```python
from build123d import *

# Parameters (mm, degrees)
SKETCH1_W                       = 10.3124
SKETCH1_H                       = 15.1892
SKETCH1_R                       = 1.8669
BOSS_EXTRUDE1_DEPTH             = 1.27
BOSS_EXTRUDE2_REACH             = 15.485
BOSS_EXTRUDE2_DIRECTION_2_REACH = 15.485
BOSS_EXTRUDE3_DEPTH             = 0.4318
LPATTERN1_COUNT                 = 5
LPATTERN1_PITCH                 = 1.27
BOSS_EXTRUDE4_DEPTH             = 6.3754
BOSS_EXTRUDE5_DEPTH             = 11.1252
BOSS_EXTRUDE5_DEPTH_BACK        = 4.7752


with BuildPart() as part:
    # Sketch1 → Boss-Extrude1 (new body)
    with BuildSketch(Plane(origin=(0, 0, 0), x_dir=(1, 0, 0), z_dir=(0, 1, 0))):
        with Locations((0, -4.8006)):
            Rectangle(SKETCH1_W, SKETCH1_H)
        with Locations(Location((0, 0, 0), (0, 0, 270))):
            Circle(SKETCH1_R, mode=Mode.SUBTRACT)
    extrude(amount=BOSS_EXTRUDE1_DEPTH)

    # Boss-Extrude2: up to this face of the body (flat: up to its plane)
    boss_extrude2_end = Plane(part.part.faces().sort_by_distance((5.1562, 0.635, 4.8006))[0])
    # Sketch2 → Boss-Extrude2 (add, up to the picked face)
    with BuildSketch(Plane(origin=(0, 0, 0), x_dir=(0, 0, -1), z_dir=(1, 0, 0)), mode=Mode.PRIVATE) as boss_extrude2_sk1:
        Polygon((-3.302, 1.2192), (-3.906625217, 4.6482), (-12.32801942, 4.6482), (-12.663922319, 2.7432), (-12.3952, 1.2192), align=None)
    boss_extrude2_tool1 = split(extrude(boss_extrude2_sk1.sketch, amount=BOSS_EXTRUDE2_REACH, mode=Mode.PRIVATE), bisect_by=boss_extrude2_end, keep=Keep.BOTH, mode=Mode.PRIVATE)
    add(boss_extrude2_tool1.solids().sort_by(Axis((0, 2.911082, 8.056355), (1, 0, 0)))[0])

    # Boss-Extrude2 direction 2: up to this face of the body (flat: up to its plane)
    boss_extrude2_direction_2_end = Plane(part.part.faces().sort_by_distance((-5.1562, 0.635, 4.8006))[0])
    # Sketch2 → Boss-Extrude2 direction 2 (add, up to the picked face)
    with BuildSketch(Plane(origin=(0, 0, 0), x_dir=(0, 0, -1), z_dir=(1, 0, 0)), mode=Mode.PRIVATE) as boss_extrude2_direction_2_sk1:
        Polygon((-3.302, 1.2192), (-3.906625217, 4.6482), (-12.32801942, 4.6482), (-12.663922319, 2.7432), (-12.3952, 1.2192), align=None)
    boss_extrude2_direction_2_tool1 = split(extrude(boss_extrude2_direction_2_sk1.sketch, amount=-BOSS_EXTRUDE2_DIRECTION_2_REACH, mode=Mode.PRIVATE), bisect_by=boss_extrude2_direction_2_end, keep=Keep.BOTH, mode=Mode.PRIVATE)
    add(boss_extrude2_direction_2_tool1.solids().sort_by(Axis((0, 2.911082, 8.056355), (-1, 0, 0)))[0])

    # Sketch3 → Boss-Extrude3 (add, symmetric)
    with BuildSketch(Plane(origin=(2.54, 0, 0), x_dir=(0, 0, -1), z_dir=(1, 0, 0))):
        with BuildLine():
            Line((-11.1252, 2.54), (-18.7452, 2.54))
            ThreePointArc((-18.7452, 2.54), (-18.762931645, 2.540154742), (-18.780657889, 2.54061892))
            Line((-18.780657889, 2.54061892), (-25.050636059, 2.759571382))
            Line((-25.050636059, 2.759571382), (-25.032907115, 3.267261922))
            Line((-25.032907115, 3.267261922), (-18.762928944, 3.04830946))
            ThreePointArc((-18.762928944, 3.04830946), (-18.754065822, 3.048077371), (-18.7452, 3.048))
            Line((-18.7452, 3.048), (-11.1252, 3.048))
            Line((-11.1252, 3.048), (-11.1252, 2.54))
        make_face()
    boss_extrude3 = extrude(amount=BOSS_EXTRUDE3_DEPTH, both=True)

    # LPattern1: Boss-Extrude3 ×5
    with Locations(*[(-i * LPATTERN1_PITCH, 0, 0) for i in range(1, LPATTERN1_COUNT)]):
        add(boss_extrude3)

    # Sketch4 → Boss-Extrude4 (add, symmetric)
    with BuildSketch(Plane(origin=(0, 0, 0), x_dir=(0, 0, -1), z_dir=(1, 0, 0))):
        Polygon((-18.796, 0.5969), (-30.48, 0.5969), (-30.48, 6.8453), (-24.2316, 6.8453), (-24.2316, 4.7371), (-17.272, 4.7371), (-17.272, 1.3589), (-18.796, 1.3589), align=None)
    extrude(amount=BOSS_EXTRUDE4_DEPTH, both=True)

    # Sketch5 → Boss-Extrude5 (add, two sides: drawn at the far end of the back side and taken through both)
    with BuildSketch(Plane.XY.offset(-BOSS_EXTRUDE5_DEPTH_BACK)):
        with BuildLine():
            Line((5.715, 0), (-5.715, 0))
            ThreePointArc((-5.715, 0), (-6.368072211, 0.237698846), (-6.715564677, 0.839573451))
            Line((-6.715564677, 0.839573451), (-9.124737032, 14.502668828))
            Line((-9.124737032, 14.502668828), (-10.125301709, 14.326242279))
            Line((-10.125301709, 14.326242279), (-7.716129354, 0.663146903))
            ThreePointArc((-7.716129354, 0.663146903), (-7.021144423, -0.540602308), (-5.715, -1.016))
            Line((-5.715, -1.016), (5.715, -1.016))
            ThreePointArc((5.715, -1.016), (7.021144423, -0.540602308), (7.716129354, 0.663146903))
            Line((7.716129354, 0.663146903), (10.125301709, 14.326242279))
            Line((10.125301709, 14.326242279), (9.124737032, 14.502668828))
            Line((9.124737032, 14.502668828), (6.715564677, 0.839573451))
            ThreePointArc((6.715564677, 0.839573451), (6.368072211, 0.237698846), (5.715, 0))
        make_face()
    extrude(amount=BOSS_EXTRUDE5_DEPTH + BOSS_EXTRUDE5_DEPTH_BACK)


solid = part.part
```
Model file for the job. Use its own axes, mm. A direction names the side the tool comes from. Round coordinates to 2 decimals unless told otherwise and drop trailing zeros. Write each loop counter-clockwise with the first axis right and the second up, starting at its lowest first coordinate (ties: lowest second). Pieces come first, ordered by that corner, then holes. Notation, with made-up numbers: M 28,37.5 L 39,37.5 A11 ccw 39,41.5 Z; hole C 29.25,-27 d9. An arc over 180 degrees is marked long. Put each result on its own line as item: value.
Item 1: Mould opens along Z. For faces 6 (the flat face through (1, 3.048, 15)), 7 (the flat face through (0.1, 2.9, 3.6)), 8 (the flat face through (-9.618, 14.416, 3.064)) say: +Z half, -Z half, draft (parallel to the pull), parting line (faces both ways), or undercut.
Responses:
face 6: undercut
face 7: -Z half
face 8: draft
Item 2: Flat gauge pins, fed straight in: P1, Ø1.5, axis at x = -6.5, y = 5, coming from the -Z side; P2, Ø1, axis at y = 2.5, z = 6, coming from the -X side; P3, Ø1, axis at y = 12, z = 4.5, coming from the -X side; P4, Ø6, axis at x = 5, y = 9, coming from the +Z side. Where does each tip first touch, or does it go through?
Responses:
P1: z = 17.27
P2: x = -8.13
P3: x = -9.8
P4: z = 30.48
Item 3: Cut at D-D (y = 8.5). List the corners of the cut face in (x, z).
Responses:
outline: M -9.1,-4.78 L -8.07,-4.78 L -8.07,11.13 L -9.1,11.13 Z; M 8.07,-4.78 L 9.1,-4.78 L 9.1,11.13 L 8.07,11.13 Z
Item 4: Cut at C-C (z = 0). List the corners of the cut face in (x, y) (3 decimals), and give its area (3 significant figures).
Responses:
outline: M -10.125,14.326 L -7.716,0.663 A2.032 ccw -5.715,-1.016 L 5.715,-1.016 A2.032 ccw 7.716,0.663 L 10.125,14.326 L 9.125,14.503 L 6.716,0.84 A1.016 cw 5.715,0 L 5.156,0 L 5.156,1.27 L 1.867,1.27 L 1.867,0 L -1.867,0 L -1.867,1.27 L -5.156,1.27 L -5.156,0 L -5.715,0 A1.016 cw -6.716,0.84 L -9.125,14.503 Z
area: 52.5 mm²
Item 5: Tool access for faces 1 (the flat face through (-5.156, 2, 7)), 2 (the flat face through (0, 0, 0)), 3 (the flat face through (0, 3.048, 15)), 4 (the flat face through (0, 4.737, 21)), 5 (the cylindrical face through (6.376, 0.244, 3.064)): list every direction of +Z, -Z, +X, -X, +Y, -Y with a clear straight run to the whole face (end or side of a thin tool).
Responses:
face 1: -Z, +Y
face 2: +Y
face 3: +X, -X, +Y
face 4: -Z, +X, -X, +Y
face 5: +Z, -Z, +Y
Item 6: Cut at B-B (x = 4.75). List the corners of the cut face in (y, z).
Responses:
outline: M -1.02,-4.78 L 0,-4.78 L 0,-2.79 L 1.27,-2.79 L 1.27,3.31 L 4.65,3.91 L 4.65,12.33 L 2.74,12.66 L 1.22,12.4 L 0,12.4 L 0,11.13 L -1.02,11.13 Z; M 0.6,18.8 L 1.36,18.8 L 1.36,17.27 L 4.74,17.27 L 4.74,24.23 L 6.85,24.23 L 6.85,30.48 L 0.6,30.48 Z
Item 7: Cut at A-A (z = 13.5). List the corners of the cut face in (x, y).
Responses:
outline: M -2.97,2.54 L -2.11,2.54 L -2.11,3.05 L -2.97,3.05 Z; M -1.7,2.54 L -0.84,2.54 L -0.84,3.05 L -1.7,3.05 Z; M -0.43,2.54 L 0.43,2.54 L 0.43,3.05 L -0.43,3.05 Z; M 0.84,2.54 L 1.7,2.54 L 1.7,3.05 L 0.84,3.05 Z; M 2.11,2.54 L 2.97,2.54 L 2.97,3.05 L 2.11,3.05 Z
Item 8: Probe L1, parallel to X at y = 1, z = 0; L2, parallel to Y at x = -1.5, z = 5; L3, parallel to Y at x = 5.25, z = 4.5. List the from-to ranges inside material, lowest first. Write a range as from..to.
Responses:
L1: -7.78..-6.74, -5.16..-1.87, 1.87..5.16, 6.74..7.78
L2: -1.02..4.65
L3: -1.02..0
